Autodesk Inventor part; units mm, degrees
ref_plane "YZ Plane" through (0, 0, 0) normal (1, 0, 0) x (0, 1, 0)
ref_plane "XZ Plane" through (0, 0, 0) normal (0, 1, 0) x (-1, 0, 0)
ref_plane "XY Plane" through (0, 0, 0) normal (0, 0, 1) x (1, 0, 0)
sketch "Sketch1" plane through (0, 0, 0) normal (0, 1, 0) x (-1, 0, 0)
  circle A0 centre (0, 0) radius 13
  dimension "d0" = 26
extrude "Extrusion1" add sketch "Sketch1" along normal blind 6
sketch "Sketch2" plane through (0, 0, 0) normal (0, -1, 0) x (1, 0, 0)
  circle A0 centre (0, 0) radius 12.5
  circle A1 centre (0, 0) radius 13
  dimension "d3" = 25
extrude "Extrusion2" cut sketch "Sketch2" against normal blind 1
sketch "Sketch3" plane through (0, 0, 0) normal (0, -1, 0) x (1, 0, 0)
  circle A0 centre (0, 0) radius 12.25
  dimension "d6" = 24.5
extrude "Extrusion3" cut sketch "Sketch3" against normal blind 5
sketch "Sketch4" plane through (0, 6, 0) normal (0, 1, 0) x (1, 0, 0)
  circle A0 centre (0, 0) radius 4
  dimension "d9" = 8
extrude "Extrusion4" add sketch "Sketch4" along normal blind 30
sketch "Sketch5" plane through (0, 36, 0) normal (0, 1, 0) x (1, 0, 0)
  circle A0 centre (0, 0) radius 4
  circle A1 centre (0, 0) radius 1
  dimension "d12" = 2
extrude "Extrusion5" cut sketch "Sketch5" against normal blind 2 contours A1
sketch "Sketch6" plane through (0, 5, 0) normal (0, -1, 0) x (1, 0, 0)
  circle A0 centre (0, 0) radius 3
  dimension "d15" = 6
extrude "Extrusion6" cut sketch "Sketch6" against normal blind 28
properties part number "Actuador"
For this review, take the finished solid that the model builds, in its own axes (mm). A direction names the side the tool comes from. Round coordinates to 2 decimals unless told otherwise and drop trailing zeros. Loops run counter-clockwise (first coordinate to the right, second up) from the corner with the lowest first, then second, coordinate; pieces in that order, holes last. Notation, with made-up numbers: (29, 72.25) - (33, 72.25) arc R21 cw to (33, 97.25) - close; hole circle Ø9 at (83, 2). An arc over 180 degrees is marked (long way). Put each result on its own line as item: value. Start each with the question number.
1. Mouldability with a two-part tool opening along X and no side actions: class faces 1 (the cylindrical face through (0, 35, 1)), 2 (the cylindrical face through (-0.867, 20.79, -3.905)), 3 (the flat face through (1, 36, 1)) as +X half, -X half, draft (parallel to the pull), parting line (faces both ways), or undercut.
2. For faces 4 (the cylindrical face through (-3, 19, 0)), 5 (the cylindrical face through (10.316, 3.465, 7.91)), 6 (the flat face through (0, 34, 0)), list the 3-axis set-ups (+Z, -Z, +X, -X, +Y, -Y) from which the entire face can be reached by the end or side of a thin tool; tool diameter is ignored.
3. Consider section A-A on z = 0. State the section outline as (x, y) points, plus the area to 4 significant figures.
4. For probe 1 along Z at (x, y) = (0, 34.7); probe 2 along Z at (x, y) = (0, 14), list the stretches that pass through material, from the lowest coordinate up. Write a range as [from, to].
5. Consider section C-C on y = 8. State the section outline as (x, z) points.
6. Consider section D-D on z = -8. State the section outline as (x, y) points, plus the area to 3 significant figures.
7. Insertion check: P1, Ø4, axis at y = 21.5, z = 1, coming from the -X side; P2, Ø2.5, axis at x = 0, z = 0, coming from the -Y side; P3, Ø6, axis at y = 6.5, z = -5, coming from the -X side. Each pin has a flat end and moves straight along its axis. Give the tip position at first contact, or say it passes through.
8. Consider section B-B on x = 0. State the section outline as (y, z) points.
Result sheet:
1. face 1: undercut
1. face 2: parting line
1. face 3: draft
2. face 4: -Y
2. face 5: +Y, -Y
2. face 6: +Y
3. outline: (-13, 1) - (-12.5, 1) - (-12.5, 0) - (-12.25, 0) - (-12.25, 5) - (-3, 5) - (-3, 33) - (3, 33) - (3, 5) - (12.25, 5) - (12.25, 0) - (12.5, 0) - (12.5, 1) - (13, 1) - (13, 6) - (4, 6) - (4, 36) - (1, 36) - (1, 34) - (-1, 34) - (-1, 36) - (-4, 36) - (-4, 6) - (-13, 6) - close
3. area: 100.5 mm^2
4. probe 1: [-4, -1], [1, 4]
4. probe 2: [-4, -3], [3, 4]
5. outline: circle Ø8 at (0, 0); hole circle Ø6 at (0, 0)
6. outline: (-10.25, 1) - (-9.6, 1) - (-9.6, 0) - (-9.28, 0) - (-9.28, 5) - (9.28, 5) - (9.28, 0) - (9.6, 0) - (9.6, 1) - (10.25, 1) - (10.25, 6) - (-10.25, 6) - close
6. area: 28.9 mm^2
7. P1: x = -4
7. P2: y = 33
7. P3: x = -12.84
8. outline: (0, -12.5) - (1, -12.5) - (1, -13) - (6, -13) - (6, -4) - (36, -4) - (36, -1) - (34, -1) - (34, 1) - (36, 1) - (36, 4) - (6, 4) - (6, 13) - (1, 13) - (1, 12.5) - (0, 12.5) - (0, 12.25) - (5, 12.25) - (5, 3) - (33, 3) - (33, -3) - (5, -3) - (5, -12.25) - (0, -12.25) - close
